Autodesk Inventor part; units mm, degrees
ref_plane "YZ Plane" through (0, 0, 0) normal (1, 0, 0) x (0, 1, 0)
ref_plane "XZ Plane" through (0, 0, 0) normal (0, 1, 0) x (-1, 0, 0)
ref_plane "XY Plane" through (0, 0, 0) normal (0, 0, 1) x (1, 0, 0)
sketch "Sketch1" plane through (0, 0, 0) normal (0, 0, 1) x (1, 0, 0)
  circle A0 centre (0, 0) radius 34.544
  dimension "d0" = 69.088
extrude "Extrusion1" add sketch "Sketch1" along normal blind 2.032
sketch "Sketch2" plane through (0, 0, 2.032) normal (0, 0, 1) x (1, 0, 0)
  line L0 (0, 0) -> (0, 29.21)
  circle A0 centre (0, 29.21) radius 1.8415
  circle A1 centre (-25.2966, 14.605) radius 1.8415
  circle A2 centre (-25.2966, -14.605) radius 1.8415
  circle A3 centre (0, -29.21) radius 1.8415
  circle A4 centre (25.2966, -14.605) radius 1.8415
  circle A5 centre (25.2966, 14.605) radius 1.8415
  dimension "d3" = 29.21
  dimension "d4" = 3.683
  dimension "d7" = 360
extrude "Extrusion2" cut sketch "Sketch2" against normal blind 2.4765
sketch "Sketch4" plane through (0, 0, 0) normal (0, 0, -1) x (-1, 0, 0)
  circle A0 centre (0, 0) radius 4.318
  dimension "d15" = 8.636
extrude "Extrusion4" cut sketch "Sketch4" against normal blind 2.4765
properties part number "pistonSealingWallFront" material "ABS Plastic"
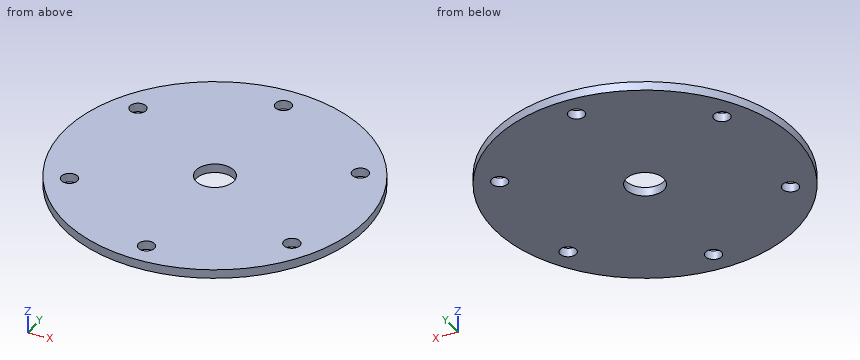
Check sheet for the modelled part. Datum: model origin and axes. Units: mm. Round coordinates to 2 decimals unless told otherwise and drop trailing zeros. Loops run counter-clockwise (first coordinate to the right, second up) from the corner with the lowest first, then second, coordinate; pieces in that order, holes last. Notation, with made-up numbers: (78, 14.5) -> (104, 14.5) arc R4 cw to (104, 21.5) -> close; hole circle Ø4 at (38, -23.5). An arc over 180 degrees is marked (long way). Answer in a Markdown table with one row per item.
Q1. Go/stop test with flat-tipped pins: P1, Ø2, axis at x = 25.3, y = -14.6, coming from the -Z side; P2, Ø11, axis at x = 0, y = 0, coming from the +Z side; P3, Ø1, axis at y = -19.5, z = 0, coming from the -X side. Record where each tip stops, or that it passes through.
Data:
| item | result |
|---|---|
| P1 | passes through |
| P2 | stops at z = 2.03 |
| P3 | stops at x = -28.85 |
Q2. Thickness scan on L1, parallel to Y at x = 0, z = 0.6; L2, parallel to Y at x = 1, z = 0.3; L3, parallel to X at y = 14.5, z = 0.45. Record the ranges inside material, lowest first.
Data:
| item | result |
|---|---|
| L1 | y = -34.54 to -31.05, -27.37 to -4.32, 4.32 to 27.37, 31.05 to 34.54 |
| L2 | y = -34.53 to -30.76, -27.66 to -4.2, 4.2 to 27.66, 30.76 to 34.53 |
| L3 | x = -31.35 to -27.14, -23.46 to 23.46, 27.14 to 31.35 |
Q3. Sectioned sample at D-D on y = -29.21. Enter the section's corners in (x, z).
Data:
| item | result |
|---|---|
| outline | (-18.44, 0) -> (-1.84, 0) -> (-1.84, 2.03) -> (-18.44, 2.03) -> close; (1.84, 0) -> (18.44, 0) -> (18.44, 2.03) -> (1.84, 2.03) -> close |
Q4. Sectioned sample at C-C on z = 1.7. Enter the section's corners in (x, y) (1 decimal).
Data:
| item | result |
|---|---|
| outline | circle Ø69.1 at (0, 0); hole circle Ø3.7 at (-25.3, -14.6); hole circle Ø3.7 at (-25.3, 14.6); hole circle Ø8.6 at (0, 0); hole circle Ø3.7 at (0, -29.2); hole circle Ø3.7 at (0, 29.2); hole circle Ø3.7 at (25.3, -14.6); hole circle Ø3.7 at (25.3, 14.6) |
Q5. Sectioned sample at B-B on x = 0. Enter the section's corners in (y, z).
Data:
| item | result |
|---|---|
| outline | (-34.54, 0) -> (-31.05, 0) -> (-31.05, 2.03) -> (-34.54, 2.03) -> close; (-27.37, 0) -> (-4.32, 0) -> (-4.32, 2.03) -> (-27.37, 2.03) -> close; (4.32, 0) -> (27.37, 0) -> (27.37, 2.03) -> (4.32, 2.03) -> close; (31.05, 0) -> (34.54, 0) -> (34.54, 2.03) -> (31.05, 2.03) -> close |
Q6. Sectioned sample at A-A on y = 0. Enter the section's corners in (x, z), then the cut area to 3 significant figures.
Data:
| item | result |
|---|---|
| outline | (-34.54, 0) -> (-4.32, 0) -> (-4.32, 2.03) -> (-34.54, 2.03) -> close; (4.32, 0) -> (34.54, 0) -> (34.54, 2.03) -> (4.32, 2.03) -> close |
| area | 123 mm^2 |
